Geometry: final body of the model. Coordinates: model frame, mm. Face numbers are marked on the shaded views. A direction names the side the tool comes from. Round coordinates to 2 decimals unless told otherwise and drop trailing zeros. Loops run counter-clockwise (first coordinate to the right, second up) from the corner with the lowest first, then second, coordinate; pieces in that order, holes last. Notation, with made-up numbers: (50, 81.25) -> (55, 81.25) arc R21 ccw to (55, 103.25) -> close; hole circle Ø8 at (-0.75, 15.25). An arc over 180 degrees is marked (long way). Answer in a Markdown table with one row per item.
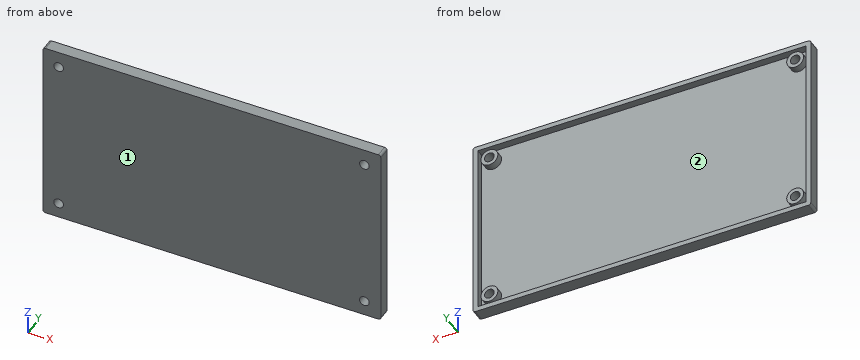
```python
from build123d import *

# Parameters (mm, degrees)
SKETCH2_W           = 139.954254508
SKETCH2_H           = 77.088138176
BOSS_EXTRUDE1_DEPTH = 2
SKETCH3_W           = 139.954254508
SKETCH3_H           = 77.088138176
SKETCH3_W_2         = 135.954254508
SKETCH3_H_2         = 73.088138176
SKETCH3_R           = 3.5
BOSS_EXTRUDE2_DEPTH = 3
SKETCH4_R           = 2
CUT_EXTRUDE1_DEPTH  = 9
FILLET1_R           = 1


with BuildPart() as part:
    # Sketch2 → Boss-Extrude1 (new body)
    with BuildSketch(Plane(origin=(0, 0, 0), x_dir=(1, 0, 0), z_dir=(0, 1, 0))):
        with Locations((67.02005334, 35.392456185)):
            Rectangle(SKETCH2_W, SKETCH2_H)
    extrude(amount=BOSS_EXTRUDE1_DEPTH)

    # Sketch3 → Boss-Extrude2 (add)
    # profile 1 of 5: a face of its own
    with BuildSketch(Plane(origin=(0, 2, 0), x_dir=(1, 0, 0), z_dir=(0, 1, 0))):
        with Locations((67.02005334, 35.392456185)):
            Rectangle(SKETCH3_W, SKETCH3_H)
        with Locations((67.02005334, 35.392456185)):
            Rectangle(SKETCH3_W_2, SKETCH3_H_2, mode=Mode.SUBTRACT)
    # profile 2 of 5: a face of its own
    with BuildSketch(Plane(origin=(0, 2, 0), x_dir=(1, 0, 0), z_dir=(0, 1, 0))):
        with Locations(Location((3.516129032, 3.642875286, 0), (0, 0, 90))):
            Circle(SKETCH3_R)
    # profile 3 of 5: a face of its own
    with BuildSketch(Plane(origin=(0, 2, 0), x_dir=(1, 0, 0), z_dir=(0, 1, 0))):
        with Locations(Location((3.516129032, 67.60985522, 0), (0, 0, 90))):
            Circle(SKETCH3_R)
    # profile 4 of 5: a face of its own
    with BuildSketch(Plane(origin=(0, 2, 0), x_dir=(1, 0, 0), z_dir=(0, 1, 0))):
        with Locations(Location((130.202184404, 67.61010922, 0), (0, 0, 90))):
            Circle(SKETCH3_R)
    # profile 5 of 5: a face of its own
    with BuildSketch(Plane(origin=(0, 2, 0), x_dir=(1, 0, 0), z_dir=(0, 1, 0))):
        with Locations(Location((130.202184404, 3.642875286, 0), (0, 0, 90))):
            Circle(SKETCH3_R)
    extrude(amount=BOSS_EXTRUDE2_DEPTH)

    # Sketch4 → Cut-Extrude1 (cut)
    with BuildSketch(Plane(origin=(0, 5, 0), x_dir=(1, 0, 0), z_dir=(0, 1, 0))):
        with Locations(Location((3.516129032, 67.60985522, 0), (0, 0, 270))):
            Circle(SKETCH4_R)
        with Locations(Location((130.202184404, 67.61010922, 0), (0, 0, 270))):
            Circle(SKETCH4_R)
        with Locations(Location((130.202184404, 3.642875286, 0), (0, 0, 270))):
            Circle(SKETCH4_R)
        with Locations(Location((3.516129032, 3.642875286, 0), (0, 0, 270))):
            Circle(SKETCH4_R)
    extrude(amount=-CUT_EXTRUDE1_DEPTH, mode=Mode.SUBTRACT)

    # Fillet1
    fillet1_edges = [part.edges().sort_by_distance(p)[0] for p in [
        (136.997180594, 2.5, -73.936525273),
        (136.997180594, 2.5, 3.151612903),
        (-2.957073914, 2.5, 3.151612903),
        (-2.957073914, 2.5, -73.936525273),
    ]]
    fillet(fillet1_edges, radius=FILLET1_R)


solid = part.part
```
Item 1: Reachability of the marked faces 1 and 2 from +Z, -Z, +X, -X, +Y, -Y: full face, straight path, thin tool, end or side. Return the list, or none.
Answer:
| item | result |
|---|---|
| face 1 | +Z, -Z, +X, -X, -Y |
| face 2 | +Y |
Item 2: Pin query (flat end, axial travel): pin 1 Ø8 at (x, z) = (43.5, -57) entering from +Y. Return the tip coordinate at first contact, or that it passes through.
Answer:
| item | result |
|---|---|
| pin 1 | stops at y = 2 |
Item 3: Cut plane C-C (x = 15). Output: boundary loops of the cut face in (y, z).
Answer:
| item | result |
|---|---|
| outline | (0, -73.94) -> (5, -73.94) -> (5, -71.94) -> (2, -71.94) -> (2, 1.15) -> (5, 1.15) -> (5, 3.15) -> (0, 3.15) -> close |
Item 4: Cut plane A-A (y = 3.95). Count the separate pieces of the cut face and the enclosed holes in it, then the cut area to 3 significant figures.
Answer:
| item | result |
|---|---|
| separate pieces | 5 |
| enclosed holes | 5 |
| area | 955 mm² |
Item 5: Cut plane D-D (z = -36.5). Output: boundary loops of the cut face in (x, y), then the cut area to 3 significant figures.
Answer:
| item | result |
|---|---|
| outline | (-2.96, 0) -> (137, 0) -> (137, 5) -> (135, 5) -> (135, 2) -> (-0.96, 2) -> (-0.96, 5) -> (-2.96, 5) -> close |
| area | 292 mm² |
Item 6: Cut plane B-B (z = -68). Output: boundary loops of the cut face in (x, y), then the cut area to 3 significant figures.
Answer:
| item | result |
|---|---|
| outline | (-2.96, 0) -> (1.55, 0) -> (1.55, 5) -> (0.04, 5) -> (0.04, 2) -> (-0.96, 2) -> (-0.96, 5) -> (-2.96, 5) -> close; (5.48, 0) -> (128.24, 0) -> (128.24, 5) -> (126.72, 5) -> (126.72, 2) -> (6.99, 2) -> (6.99, 5) -> (5.48, 5) -> close; (132.16, 0) -> (137, 0) -> (137, 5) -> (135, 5) -> (135, 2) -> (133.68, 2) -> (133.68, 5) -> (132.16, 5) -> close |
| area | 294 mm² |
Item 7: Line query: probe 1 along X at (y, z) = (2.65, -12.5); probe 2 along Z at (x, y) = (108, 4.3); probe 3 along X at (y, z) = (4.2, -2.5). Output: solid intervals per line, ascending. Write a range as [from, to].
Answer:
| item | result |
|---|---|
| probe 1 | x = [-2.96, -0.96], [135, 137] |
| probe 2 | z = [-73.94, -71.94], [1.15, 3.15] |
| probe 3 | x = [-2.96, -0.96], [0.21, 1.87], [5.16, 6.82], [126.89, 128.56], [131.84, 133.51], [135, 137] |
